Check sheet for the modelled part. Datum: model origin and axes. Units: mm. Round coordinates to 2 decimals unless told otherwise and drop trailing zeros. Write each loop counter-clockwise with the first axis right and the second up, starting at its lowest first coordinate (ties: lowest second). Pieces come first, ordered by that corner, then holes.
Item 1: Material ranges on line 1 (Z direction, x = 0, y = -0.8); line 2 (X direction, y = -1.6, z = 0.5); line 3 (Z direction, x = -15, y = -1.1), recorded low to high.
Item 2: Cross-section at C-C on x = 15. Enter the section's corners in (y, z).
Item 3: Cross-section at D-D on z = -20. Enter the section's corners in (x, y), plus the area to 3 significant figures.
Item 4: Cross-section at A-A on z = 0. Enter the section's corners in (x, y).
Item 5: Cross-section at B-B on y = -0.9. Count the separate pieces of the cut face and the enclosed holes in it, plus the area to 3 significant figures.
Item 6: Go/stop test with flat-tipped pins: pin 1 Ø2 at (x, z) = (-15, -15) entering from -Y; pin 2 Ø0.6 at (y, z) = (-0.5, -33) entering from -X; pin 3 Ø1 at (y, z) = (-1, -32.5) entering from +X. Record where each tip stops, or that it passes through.
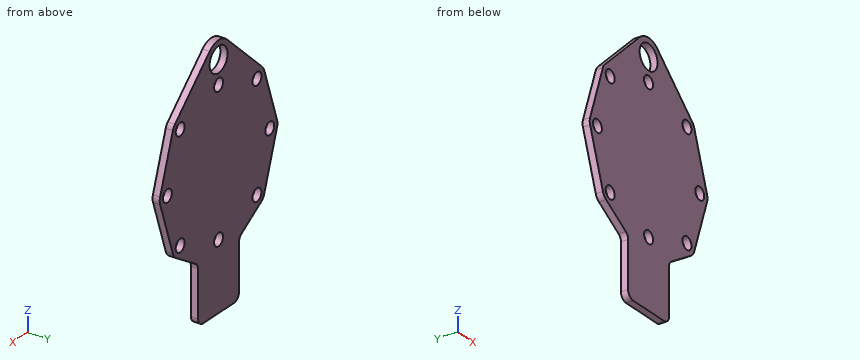
from build123d import *

# Parameters (mm, degrees)
F0_R     = 1.75
F0_R_2   = 3.5
F1_DEPTH = 2


with BuildPart() as f1:
    # F0 (on Front) → F1 (new body)
    with BuildSketch(Plane.XZ):
        with BuildLine():
            Line((8.927711, -22.410767), (16.608433, -17.532379))
            ThreePointArc((16.608433, -17.532379), (17.363816, -16.847261), (17.84605, -15.948683))
            Line((17.84605, -15.948683), (22.84605, -0.948683))
            ThreePointArc((22.84605, -0.948683), (23, 0), (22.84605, 0.948683))
            Line((22.84605, 0.948683), (17.84605, 15.948683))
            ThreePointArc((17.84605, 15.948683), (17.531795, 16.609352), (17.066972, 17.174311))
            Line((17.066972, 17.174311), (3.444953, 30.123852))
            ThreePointArc((3.444953, 30.123852), (0, 31.5), (-3.444953, 30.123852))
            Line((-3.444953, 30.123852), (-17.066972, 17.174311))
            ThreePointArc((-17.066972, 17.174311), (-17.531795, 16.609352), (-17.84605, 15.948683))
            Line((-17.84605, 15.948683), (-22.84605, 0.948683))
            ThreePointArc((-22.84605, 0.948683), (-23, 0), (-22.84605, -0.948683))
            Line((-22.84605, -0.948683), (-17.84605, -15.948683))
            ThreePointArc((-17.84605, -15.948683), (-17.363816, -16.847261), (-16.608433, -17.532379))
            Line((-16.608433, -17.532379), (-8.927711, -22.410767))
            ThreePointArc((-8.927711, -22.410767), (-8.247205, -23.135842), (-8, -24.09902))
            Line((-8, -24.09902), (-8, -37))
            ThreePointArc((-8, -37), (-7.414214, -38.414214), (-6, -39))
            Line((-6, -39), (6, -39))
            ThreePointArc((6, -39), (7.414214, -38.414214), (8, -37))
            Line((8, -37), (8, -24.09902))
            ThreePointArc((8, -24.09902), (8.247205, -23.135842), (8.927711, -22.410767))
        make_face()
        with Locations((-15, -15)):
            Circle(F0_R, mode=Mode.SUBTRACT)
        with Locations((0, -20)):
            Circle(F0_R, mode=Mode.SUBTRACT)
        with Locations((15, -15)):
            Circle(F0_R, mode=Mode.SUBTRACT)
        with Locations((-20, 0)):
            Circle(F0_R, mode=Mode.SUBTRACT)
        with Locations((-15, 15)):
            Circle(F0_R, mode=Mode.SUBTRACT)
        with Locations((20, 0)):
            Circle(F0_R, mode=Mode.SUBTRACT)
        with Locations((0, 20)):
            Circle(F0_R, mode=Mode.SUBTRACT)
        with Locations((0, 26.5)):
            Circle(F0_R_2, mode=Mode.SUBTRACT)
        with Locations((15, 15)):
            Circle(F0_R, mode=Mode.SUBTRACT)
    extrude(amount=F1_DEPTH)


solid = f1.part
Response values:
1. line 1: z = -39 to -21.75, -18.25 to 18.25, 21.75 to 23, 30 to 31.5
1. line 2: x = -22.96 to -21.68, -18.32 to 18.32, 21.68 to 22.96
1. line 3: z = -18.55 to -16.75, -13.25 to 13.25, 16.75 to 19.14
2. outline: (-2, -18.55) - (0, -18.55) - (0, -16.75) - (-2, -16.75) - close; (-2, -13.25) - (0, -13.25) - (0, 13.25) - (-2, 13.25) - close; (-2, 16.75) - (0, 16.75) - (0, 19.14) - (-2, 19.14) - close
3. outline: (-12.72, -2) - (-1.75, -2) - (-1.75, 0) - (-12.72, 0) - close; (1.75, -2) - (12.72, -2) - (12.72, 0) - (1.75, 0) - close
3. area: 43.9 mm2
4. outline: (-23, -2) - (-21.75, -2) - (-21.75, 0) - (-23, 0) - close; (-18.25, -2) - (18.25, -2) - (18.25, 0) - (-18.25, 0) - close; (21.75, -2) - (23, -2) - (23, 0) - (21.75, 0) - close
5. separate pieces: 1
5. enclosed holes: 9
5. area: 1,950 mm2
6. pin 1: passes through
6. pin 2: stops at x = -8
6. pin 3: stops at x = 8
